Part model, mm, in its own coordinate system. A direction names the side the tool comes from. Give positions to 0.01 mm unless a question says otherwise; leave off trailing zeros. Write each loop counter-clockwise with the first axis right and the second up, starting at its lowest first coordinate (ties: lowest second). Pieces come first, ordered by that corner, then holes. Notation, with made-up numbers: (65, 11) - (72, 11) arc R22 ccw to (72, 49) - close; hole circle Ø7 at (-3, 72). An arc over 180 degrees is marked (long way). Answer as a JSON object with one key per item and string values. Group by question number.
```python
from build123d import *

# Parameters (mm, degrees)
F0_W          = 25.4
F0_H          = 25.4
F1_DEPTH      = 254
F1_DEPTH_BACK = 254
F3_D          = 3.6068
F6_D          = 12.7
F7_D          = 6.35
F7_DEPTH      = 3.175
F7_TIP        = 1.9077324654
F8_W          = 25.4
F8_H          = 25.4
F8_R          = 6.35
F9_DEPTH      = 101.6
F10_W         = 25.4
F10_H         = 25.4
F10_R         = 6.35
F11_DEPTH     = 101.6
F12_W         = 203.2
F12_H         = 25.4
F13_DEPTH     = 25.4


with BuildPart() as f1:
    # F0 (on Right) → F1 (new body, two sides)
    with BuildSketch(Plane.YZ) as f1_sk:
        Polygon((-57.15, -25.4), (-57.15, 0), (-31.75, 0), (31.75, 0), (57.15, 0), (57.15, -25.4), (63.5, -25.4), (63.5, 6.35), (-63.5, 6.35), (-63.5, -25.4), align=None)
        with Locations((-44.45, -12.7)):
            Rectangle(F0_W, F0_H)
        with Locations((44.45, -12.7)):
            Rectangle(F0_W, F0_H)
    extrude(amount=F1_DEPTH)
    extrude(f1_sk.sketch, amount=-F1_DEPTH_BACK)

    # F3 (through all)
    with Locations(Plane.XY.offset(6.35)):
        with Locations((-226.6823, 0), (-201.4855, 0), (-176.2887, 0), (-151.0919, 0), (-125.7427, 0), (-100.9523, 0), (-75.5523, 0), (-50.5333, 0), (-25.3873, 0), (-0.0635, 0), (25.0825, 0), (50.3809, 0), (72.2249, 0), (94.3483, 0), (116.4971, 0), (138.1379, 0), (160.4137, 0), (182.6641, 0), (204.4065, 0), (226.6823, 0)):
            Hole(F3_D / 2)

    # F6 (through all)
    with Locations(Plane.YZ.offset(254)):
        with Locations((-44.45, -12.7), (44.45, -12.7)):
            Hole(F6_D / 2)

    # F7
    with Locations(Plane.XZ.offset(63.5)):
        with Locations((-226.6823, -12.7), (-201.4855, -12.7), (-176.2887, -12.7), (-151.0919, -12.7), (-125.7427, -12.7), (-100.9523, -12.7), (-75.5523, -12.7), (-50.5333, -12.7), (-25.3873, -12.7), (-0.0635, -12.7), (25.0825, -12.7), (50.3809, -12.7), (72.2249, -12.7), (94.3483, -12.7), (116.4971, -12.7), (138.1379, -12.7), (160.4137, -12.7), (182.6641, -12.7), (204.4065, -12.7), (226.6823, -12.7)):
            Hole(F7_D / 2, depth=F7_DEPTH)
            with Locations((0, 0, -(F7_DEPTH + F7_TIP / 2))):  # 118° drill point
                Cone(0, F7_D / 2, F7_TIP, mode=Mode.SUBTRACT)

    # F8 (on face) → F9 (cut)
    with BuildSketch(Plane.YZ.offset(254)):
        with Locations((44.45, -12.7)):
            Rectangle(F8_W, F8_H)
        with Locations((44.45, -12.7)):
            Circle(F8_R, mode=Mode.SUBTRACT)
        with Locations((-44.45, -12.7)):
            Rectangle(F8_W, F8_H)
        with Locations((-44.45, -12.7)):
            Circle(F8_R, mode=Mode.SUBTRACT)
    extrude(amount=-F9_DEPTH, mode=Mode.SUBTRACT)

    # F10 (on face) → F11 (cut)
    with BuildSketch(Plane(origin=(-254, 0, 0), x_dir=(0, -1, 0), z_dir=(-1, 0, 0))):
        with Locations((-44.45, -12.7)):
            Rectangle(F10_W, F10_H)
        with Locations((-44.45, -12.7)):
            Circle(F10_R, mode=Mode.SUBTRACT)
        with Locations((44.45, -12.7)):
            Rectangle(F10_W, F10_H)
        with Locations((44.45, -12.7)):
            Circle(F10_R, mode=Mode.SUBTRACT)
    extrude(amount=-F11_DEPTH, mode=Mode.SUBTRACT)

    # F12 (on face) → F13 (cut)
    with BuildSketch(Plane(origin=(0, 0, -25.4), x_dir=(1, 0, 0), z_dir=(0, 0, -1))):
        with Locations((0, -44.45)):
            Rectangle(F12_W, F12_H)
        with Locations((0, 44.45)):
            Rectangle(F12_W, F12_H)
    extrude(amount=-F13_DEPTH, mode=Mode.SUBTRACT)


solid = f1.part
```
1) Drill centre lines: line 1 along Y through (x, z) = (-92.5, -16.5); line 2 along X through (y, z) = (49.5, -21.5); line 3 along Y through (x, z) = (-112, -23.5). Where is each one in solid material? Low to high. Write a range as from..to.
2) Two-plate mould, pull along X, no slides. Class faces 5 (the flat face through (152.4, 38.6, -9.7)), 6 (the flat face through (204, 57.15, -13)), 7 (the flat face through (101.6, 47, -19)), 8 (the flat face through (-152.4, -38.6, -9.7)): +X half, -X half, draft (parallel to the pull), parting line (faces both ways), or undercut.
3) Saw through at A-A (y = -44.45). List the corners of the cut face in (x, z).
4) Which spindle directions (+Z, -Z, +X, -X, +Y, -Y) get a long thin tool onto all of the face, cutting with end or side? Do faces 1 (the flat face through (-204, 57.15, -13)), 2 (the flat face through (-101.6, -38.6, -15.7)), 3 (the flat face through (-127, 31.75, -13)), 4 (the cylindrical face through (126.644, -50.316, -15.132)). Say none if no direction does.
5) Drop flat-ended pins along their axis: P1, Ø4.5, axis at x = -25.39, y = 0, coming from the -Z side; P2, Ø12.5, axis at y = 48.5, z = -7.5, coming from the +X side; P3, Ø3, axis at y = 29, z = -3, coming from the +X side; P4, Ø5.5, axis at x = 160.41, z = -12.7, coming from the -Y side. Give the stop position or say it passes through.
Checks:
{
 "1": {"line 1": "-63.5..-57.15, 57.15..63.5", "line 2": "-152.4..-101.6, 101.6..152.4", "line 3": "-63.5..-31.75, 31.75..63.5"},
 "2": {"face 5": "+X half", "face 6": "draft", "face 7": "undercut", "face 8": "-X half"},
 "3": {"outline": "(-254, 0) - (-152.4, 0) - (-152.4, -6.35) - (-101.6, -6.35) - (-101.6, 0) - (101.6, 0) - (101.6, -6.35) - (152.4, -6.35) - (152.4, 0) - (254, 0) - (254, 6.35) - (-254, 6.35) - close; (-152.4, -25.4) - (-101.6, -25.4) - (-101.6, -19.05) - (-152.4, -19.05) - close; (101.6, -25.4) - (152.4, -25.4) - (152.4, -19.05) - (101.6, -19.05) - close"},
 "4": {"face 1": "-Z, -X", "face 2": "-Z", "face 3": "-Z, +X, -X", "face 4": "+X, -X"},
 "5": {"P1": "z = 0", "P2": "x = 152.4", "P3": "through", "P4": "y = -60.07"}
}
